Geometry: final body of the model. Coordinates: model frame, mm. A direction names the side the tool comes from. Coordinates: 2 decimals unless noted, no trailing zeros. Write each loop counter-clockwise with the first axis right and the second up, starting at its lowest first coordinate (ties: lowest second). Pieces come first, ordered by that corner, then holes.
Autodesk Inventor part; units mm, degrees
ref_plane "Start Plane" through (0, 0, 10) normal (0, 0, 1) x (1, 0, 0)
ref_plane "End Plane" through (0, 0, 300) normal (0, 0, 1) x (1, 0, 0)
ref_plane "Work Plane4" through (155, -7, 300) normal (0, 0, 1) x (1, 0, 0)
ref_plane "Start Plane" through (0, 0, 10) normal (0, 0, 1) x (1, 0, 0)
ref_plane "End Plane" through (0, 0, 300) normal (0, 0, 1) x (1, 0, 0)
sketch "Sketch" plane through (0, 0, 0) normal (0, 0, 1) x (1, 0, 0)
  line L0 (-10, -7) -> (-10, 7)
  line L1 (-7, 10) -> (7, 10)
  line L2 (10, 7) -> (10, -7)
  line L3 (7, -10) -> (-7, -10)
  arc A0 (-10, -7) -> (-7, -10) centre (-7, -7) ccw
  arc A1 (-7, 10) -> (-10, 7) centre (-7, 7) ccw
  arc A2 (10, 7) -> (7, 10) centre (7, 7) ccw
  arc A3 (7, -10) -> (10, -7) centre (7, -7) ccw
  arc A4 (-7, 8) -> (-8, 7) centre (-7, 7) ccw
  line L4 (-7, 8) -> (7, 8)
  arc A5 (8, 7) -> (7, 8) centre (7, 7) ccw
  line L5 (8, 7) -> (8, -7)
  arc A6 (7, -8) -> (8, -7) centre (7, -7) ccw
  line L6 (7, -8) -> (-7, -8)
  arc A7 (-8, -7) -> (-7, -8) centre (-7, -7) ccw
  line L7 (-8, -7) -> (-8, 7)
  line L8 (0, 14.8698) -> (0, -14.8698) construction
  line L9 (-14.8698, 0) -> (14.8698, 0) construction
  dimension "d7" = 3
  dimension "d10" = 20
  dimension "d11" = 20
  dimension "d12" = 2
  dimension "d15" = 10
  dimension "d16" = 10
extrude "Body" add sketch "Sketch" along normal up to surface (290 mm away) from surface at 10
sketch "Sketch3" plane through (0, 0, 0) normal (0, 0, 1) x (1, 0, 0)
  line L0 (0, 0) -> (10, 0)
ref_plane "Work Plane3" through (0, 0, 0) normal (0, -1, 0) x (1, 0, 0)
sketch "Sketch4" plane through (0, 0, 0) normal (0, -1, 0) x (1, 0, 0)
  line L0 (-2, 10) -> (12, 10)
  line L1 (-2, 300) -> (12, 300)
  dimension "d18" = 290
ref_plane "Work Plane4" through (155, -7, 300) normal (0, 0, 1) x (1, 0, 0)
split "Split1" plane through (155, -7, 300) removes the side toward (0, 0, 1)
ref_plane "Work Plane5" through (-75, -7, 10) normal (0, 0, -1) x (-1, 0, 0)
split "Split2" plane through (-75, -7, 10) removes the side toward (0, 0, -1)
equation "\"d7\" = G_IR"
equation "\"d10\" = G_H"
equation "\"d11\" = G_W"
equation "\"d12\" = G_T"
equation "\"d15\" = 0.5 * d10"
equation "\"d16\" = 0.5 * d11"
equation "\"d3\" = G_L"
equation "\"G_W\" = 20"
equation "\"G_H\" = 20"
equation "\"G_T\" = 2"
equation "\"G_IR\" = 3"
equation "\"G_L\" = d18"
properties part number "ISO 12633-2 - 20x20x2 - 290" material "Steel, Mild"
Item 1: Material intervals for probe 1 along X at (y, z) = (-1.5, 199.5); probe 2 along X at (y, z) = (-7.5, 218), sorted ascending.
Derived:
probe 1: x = -10 to -8, 8 to 10
probe 2: x = -9.96 to -7.87, 7.87 to 9.96
Item 2: Section C-C, the plane z = 52. Output: boundary loops of the cut face in (x, y), plus the area to 3 significant figures.
Derived:
outline: (-10, -7) arc R3 ccw to (-7, -10) - (7, -10) arc R3 ccw to (10, -7) - (10, 7) arc R3 ccw to (7, 10) - (-7, 10) arc R3 ccw to (-10, 7) - close; hole (-8, -7) arc R1 ccw to (-7, -8) - (7, -8) arc R1 ccw to (8, -7) - (8, 7) arc R1 ccw to (7, 8) - (-7, 8) arc R1 ccw to (-8, 7) - close
area: 137 mm2
Item 3: Set-up query: faces 1 (the flat face through (0, 8, 153)), 2 (the flat face through (-9, 0, 10)). Return all of +Z, -Z, +X, -X, +Y, -Y with unobstructed straight access to the full face (end or side cutting, diameter ignored); none if empty.
Derived:
face 1: +Z, -Z
face 2: -Z, +X, -X, +Y, -Y
Item 4: Pull-direction query (X, two-part tool) for faces 3 (the flat face through (0, -8, 153)), 4 (the flat face through (0, 10, 153)), 5 (the flat face through (10, 0, 153)); classes: released by +X, released by -X, zero draft, split by the parting line, or undercut.
Derived:
face 3: undercut
face 4: zero draft
face 5: released by +X
Item 5: Pin query (flat end, axial travel): pin 1 (5 mm diameter, centred on x = -3.5, y = -2.5, fed in from -Z). Return the tip coordinate at first contact, or that it passes through.
Derived:
pin 1: passes through
Item 6: Section A-A, the plane x = 2. Output: boundary loops of the cut face in (y, z).
Derived:
outline: (-10, 10) - (-8, 10) - (-8, 300) - (-10, 300) - close; (8, 10) - (10, 10) - (10, 300) - (8, 300) - close
